The model under review builds one solid part; all positions refer to its coordinate system, in mm. Coordinates: 2 decimals unless noted, no trailing zeros. Write each loop counter-clockwise with the first axis right and the second up, starting at its lowest first coordinate (ties: lowest second). Pieces come first, ordered by that corner, then holes. Notation, with made-up numbers: (-23.75, 78.25) -> (-17.75, 78.25) arc R32 cw to (-17.75, 105.25) -> close; hole circle Ø10 at (85, -36). An arc over 180 degrees is marked (long way). Write each question's results on one line, items separated by ' | '.
Solid Edge part; units mm, degrees
sketch "Sketch1" plane through (0, 66.5, 0) normal (0, 1, 0) x (-1, 0, 0)
  circle A0 centre (13.0488, 5.0062) radius 1.7126
  line L0 (20.5735, 0.0023) -> (20.5735, 10)
  line L1 (20.5735, 10) -> (-9.472, 10)
  line L2 (-9.472, 10) -> (-9.472, 0.0023)
  line L3 (-9.472, 0.0023) -> (20.5735, 0.0023)
  circle A1 centre (-1.9473, 4.9961) radius 1.7148
extrude "Protrusion1" add sketch "Sketch1" along normal blind 5
sketch "Sketch2" plane through (-5.5507, 69, 0.0023) normal (0, 0, -1) x (1, 0, 0)
  arc A0 (3.6559, 2.5) -> (0.4426, 2.5) centre (2.0493, 2.5) cw
  line L0 (3.6559, 2.5) -> (0.4426, 2.5)
  arc A1 (-0.3116, 2.5) -> (-3.5939, 2.5) centre (-1.9527, 2.5) cw
  line L1 (-0.3116, 2.5) -> (-3.5939, 2.5)
extrude "ExtrudedCutout_1" cut sketch "Sketch2" against normal blind 32
fillet "Round_1" radius 2 3 edges at (9.472, 71.5, 5.0011) (-20.5735, 71.5, 5.0011) (-5.5507, 71.5, 10)
Q1. Add section C-C (x = 1.5). Write out the cut boundary in (y, z), plus the area to 3 significant figures.
Solution:
outline: (66.5, 0) -> (71.5, 0) -> (71.5, 3.34) -> (66.5, 3.34) -> close; (66.5, 6.65) -> (71.5, 6.65) -> (71.5, 8) arc R2 ccw to (69.5, 10) -> (66.5, 10) -> close | area: 32.6 mm²
Q2. Clearance check with a flat-ended pin moving along its axis: P1, Ø2, axis at x = -13.05, z = 5.01, coming from the -Y side. State where the tip first meets the part, or that it passes through.
Solution:
P1: through
Q3. Add section B-B (z = 4.25). Write out the cut boundary in (x, y), plus the area to 3 significant figures.
Solution:
outline: (-20.57, 66.5) -> (-14.59, 66.5) -> (-14.59, 71.5) -> (-18.57, 71.5) arc R2 ccw to (-20.57, 69.5) -> close; (-11.51, 66.5) -> (-9.14, 66.5) arc R1.64 cw to (-5.86, 66.5) -> (-5.11, 66.5) arc R1.61 cw to (-1.89, 66.5) -> (0.4, 66.5) -> (0.4, 71.5) -> (-11.51, 71.5) -> close; (3.49, 66.5) -> (9.47, 66.5) -> (9.47, 69.5) arc R2 ccw to (7.47, 71.5) -> (3.49, 71.5) -> close | area: 109 mm²
Q4. Add section D-D (x = 6.5). Write out the cut boundary in (y, z), plus the area to 3 significant figures.
Solution:
outline: (66.5, 0) -> (71.5, 0) -> (71.5, 8) arc R2 ccw to (69.5, 10) -> (66.5, 10) -> close | area: 49.1 mm²
Q5. Draft analysis for pull direction X (two halves, no side actions). For faces 1 (the flat face through (9.472, 68, 5)), 2 (the cylindrical face through (-3.537, 68.106, 4.931)), 3 (the flat face through (-20.574, 68, 5)), 4 (the flat face through (-15, 66.5, 5)), state which applies: pulls with the +X half, pulls with the -X half, needs draft (parallel to the pull), parting line crosses it, or undercut.
Solution:
face 1: pulls with the +X half | face 2: undercut | face 3: pulls with the -X half | face 4: needs draft
Q6. Add section A-A (y = 67.25). Write out the cut boundary in (x, z).
Solution:
outline: (-20.57, 0) -> (-8.96, 0) -> (-8.96, 10) -> (-20.57, 10) -> close; (-6.04, 0) -> (-4.92, 0) -> (-4.92, 10) -> (-6.04, 10) -> close; (-2.08, 0) -> (9.47, 0) -> (9.47, 10) -> (-2.08, 10) -> close; hole circle Ø3.43 at (-13.05, 5.01); hole circle Ø3.43 at (1.95, 5)
Q7. For line 1 (X direction, y = 67.4, z = 2.75); line 2 (Z direction, x = 2, y = 67.8); line 3 (X direction, y = 67.65, z = 2), list the stretches that pass through material, from the lowest coordinate up. Write a range as from..to.
Solution:
line 1: -20.57..-8.88, -6.13..-4.83, -2.17..9.47 | line 2: 0..3.28, 6.71..10 | line 3: -20.57..-8.67, -6.33..-4.62, -2.38..9.47
